Here's how the part is built. I have some questions about the finished solid (model axes, mm). A direction names the side the tool comes from. Coordinates: 2 decimals unless noted, no trailing zeros. Loops run counter-clockwise (first coordinate to the right, second up) from the corner with the lowest first, then second, coordinate; pieces in that order, holes last. Notation, with made-up numbers: (-20, 14.5) - (18, 14.5) arc R6 cw to (18, 23.5) - close; hole circle Ø5 at (2.5, 67.5). An arc over 180 degrees is marked (long way). Use a Markdown table: item, result.
```python
from build123d import *

# Parameters (mm, degrees)
SKETCH_1_W          = 8
SKETCH_1_H          = 8
SKETCH_1_W_2        = 6
SKETCH_1_H_2        = 6
EXTRUDE_1_DEPTH     = 50
FILLET_1_R          = 0.2
FILLET_2_R          = 0.2
SKETCH_3_R          = 1.65
CUT_EXTRUDE_1_DEPTH = 50
SKETCH_4_R          = 1.65
CUT_EXTRUDE_2_DEPTH = 50


with BuildPart() as part:
    # 草图1 → 凸台-拉伸1 (new body)
    with BuildSketch(Plane(origin=(0, 0, 0), x_dir=(1, 0, 0), z_dir=(0, 1, 0))):
        Rectangle(SKETCH_1_W, SKETCH_1_H)
        Rectangle(SKETCH_1_W_2, SKETCH_1_H_2, mode=Mode.SUBTRACT)
    extrude(amount=EXTRUDE_1_DEPTH)

    # 圆角1
    fillet_1_edges = [part.edges().sort_by_distance(p)[0] for p in [
        (3, 25, 3),
        (3, 25, -3),
        (-3, 25, -3),
        (-3, 25, 3),
    ]]
    fillet(fillet_1_edges, radius=FILLET_1_R)

    # 圆角2
    fillet_2_edges = [part.edges().sort_by_distance(p)[0] for p in [
        (4, 25, 4),
        (-4, 25, 4),
        (-4, 25, -4),
        (4, 25, -4),
    ]]
    fillet(fillet_2_edges, radius=FILLET_2_R)

    # 草图3 → 切除-拉伸1 (cut)
    with BuildSketch(Plane(origin=(4, 0, 0), x_dir=(0, 0, -1), z_dir=(1, 0, 0))):
        with Locations((0, 39)):
            Circle(SKETCH_3_R)
        with Locations((0, 11)):
            Circle(SKETCH_3_R)
    extrude(amount=-CUT_EXTRUDE_1_DEPTH, mode=Mode.SUBTRACT)

    # 草图4 → 切除-拉伸2 (cut)
    with BuildSketch(Plane(origin=(0, 0, -4), x_dir=(-1, 0, 0), z_dir=(0, 0, -1))):
        with Locations((0, 44)):
            Circle(SKETCH_4_R)
        with Locations((0, 6)):
            Circle(SKETCH_4_R)
    extrude(amount=-CUT_EXTRUDE_2_DEPTH, mode=Mode.SUBTRACT)


solid = part.part
```
Q1. I want a section at D-D, the plane y = 19.5. Write out the boundary of the cut face in (x, z), then the cut area to 3 significant figures.
Check values:
| item | result |
|---|---|
| outline | (-4, -3.8) arc R0.2 ccw to (-3.8, -4) - (3.8, -4) arc R0.2 ccw to (4, -3.8) - (4, 3.8) arc R0.2 ccw to (3.8, 4) - (-3.8, 4) arc R0.2 ccw to (-4, 3.8) - close; hole (-3, -2.8) arc R0.2 ccw to (-2.8, -3) - (2.8, -3) arc R0.2 ccw to (3, -2.8) - (3, 2.8) arc R0.2 ccw to (2.8, 3) - (-2.8, 3) arc R0.2 ccw to (-3, 2.8) - close |
| area | 28.0 mm^2 |
Q2. I want a section at A-A, the plane z = 0. Write out the boundary of the cut face in (x, y).
Check values:
| item | result |
|---|---|
| outline | (-4, 0) - (-3, 0) - (-3, 9.35) - (-4, 9.35) - close; (-4, 12.65) - (-3, 12.65) - (-3, 37.35) - (-4, 37.35) - close; (-4, 40.65) - (-3, 40.65) - (-3, 50) - (-4, 50) - close; (3, 0) - (4, 0) - (4, 9.35) - (3, 9.35) - close; (3, 12.65) - (4, 12.65) - (4, 37.35) - (3, 37.35) - close; (3, 40.65) - (4, 40.65) - (4, 50) - (3, 50) - close |
Q3. If we mould it in two halves opening along X, with no side actions, what happens to faces 3 (the face through (0.4, 4.4, 3.5)), 4 (the face through (0, 25, 4)), 5 (the face through (4, 25, 0))? For each: pulls with the +X half, pulls with the -X half, needs draft (parallel to the pull), parting line crosses it, or undercut.
Check values:
| item | result |
|---|---|
| face 3 | undercut |
| face 4 | needs draft |
| face 5 | pulls with the +X half |
Q4. I want a section at B-B, the plane y = 6. Write out the boundary of the cut face in (x, z).
Check values:
| item | result |
|---|---|
| outline | (-4, -3.8) arc R0.2 ccw to (-3.8, -4) - (-1.65, -4) - (-1.65, -3) - (-2.8, -3) arc R0.2 cw to (-3, -2.8) - (-3, 2.8) arc R0.2 cw to (-2.8, 3) - (-1.65, 3) - (-1.65, 4) - (-3.8, 4) arc R0.2 ccw to (-4, 3.8) - close; (1.65, -4) - (3.8, -4) arc R0.2 ccw to (4, -3.8) - (4, 3.8) arc R0.2 ccw to (3.8, 4) - (1.65, 4) - (1.65, 3) - (2.8, 3) arc R0.2 cw to (3, 2.8) - (3, -2.8) arc R0.2 cw to (2.8, -3) - (1.65, -3) - close |
Q5. Please list where these lines run through material, in increasing order: L1, parallel to Y at x = 0, z = 3.5; L2, parallel to Z at x = 2, y = 25.5. Write a range as from..to.
Check values:
| item | result |
|---|---|
| L1 | 0..4.35, 7.65..42.35, 45.65..50 |
| L2 | -4..-3, 3..4 |
Q6. Which directions (+Z, -Z, +X, -X, +Y, -Y) give clear straight access to the entire face, cutting with the end or side of a thin tool? Please do faces 1 (the face through (3.5, 0, -0.1)), 2 (the face through (-3, 25, 0)).
Check values:
| item | result |
|---|---|
| face 1 | +Z, -Z, +X, -X, -Y |
| face 2 | +Y, -Y |
Q7. I want a section at C-C, the plane x = 0. Write out the boundary of the cut face in (y, z).
Check values:
| item | result |
|---|---|
| outline | (0, -4) - (4.35, -4) - (4.35, -3) - (0, -3) - close; (0, 3) - (4.35, 3) - (4.35, 4) - (0, 4) - close; (7.65, -4) - (42.35, -4) - (42.35, -3) - (7.65, -3) - close; (7.65, 3) - (42.35, 3) - (42.35, 4) - (7.65, 4) - close; (45.65, -4) - (50, -4) - (50, -3) - (45.65, -3) - close; (45.65, 3) - (50, 3) - (50, 4) - (45.65, 4) - close |
